```python
from build123d import *

# Parameters (mm, degrees)
SKETCH_1_R          = 80
EXTRUDE_1_DEPTH     = 10
SKETCH_2_R          = 10
CUT_EXTRUDE_1_DEPTH = 10
SKETCH_3_R          = 45
EXTRUDE_2_DEPTH     = 140
SKETCH_6_R          = 10
CUT_EXTRUDE_3_DEPTH = 181
SKETCH_7_R          = 30
SKETCH_7_R_2        = 15
EXTRUDE_3_DEPTH     = 60
SKETCH_8_R          = 15
CUT_EXTRUDE_4_DEPTH = 45
SKETCH_9_R          = 10
CUT_EXTRUDE_5_DEPTH = 200
FILLET_1_R          = 2


with BuildPart() as part:
    # 草图1 → 凸台-拉伸1 (new body)
    with BuildSketch(Plane.XY):
        Circle(SKETCH_1_R)
    extrude(amount=EXTRUDE_1_DEPTH)

    # 草图2 → 切除-拉伸1 (cut)
    with BuildSketch(Plane.XY):
        with Locations((32.5, 56.291651246)):
            Circle(SKETCH_2_R)
        with Locations((-32.5, -56.291651246)):
            Circle(SKETCH_2_R)
        with Locations((-65, 0)):
            Circle(SKETCH_2_R)
        with Locations((-32.5, 56.291651246)):
            Circle(SKETCH_2_R)
        with Locations((65, 0)):
            Circle(SKETCH_2_R)
        with Locations((32.5, -56.291651246)):
            Circle(SKETCH_2_R)
    extrude(amount=CUT_EXTRUDE_1_DEPTH, mode=Mode.SUBTRACT)

    # 草图3 → 凸台-拉伸2 (add)
    with BuildSketch(Plane.XY):
        Circle(SKETCH_3_R)
    extrude(amount=-EXTRUDE_2_DEPTH)

    # 草图6 → 切除-拉伸3 (cut, through all)
    with BuildSketch(Plane.XY):
        Circle(SKETCH_6_R)
    extrude(amount=-CUT_EXTRUDE_3_DEPTH, mode=Mode.SUBTRACT)

    # 草图7 → 凸台-拉伸3 (add)
    with BuildSketch(Plane(origin=(0, 0, 0), x_dir=(0, 0, -1), z_dir=(1, 0, 0))):
        with Locations((110, 0)):
            Circle(SKETCH_7_R)
        with Locations((110, 0)):
            Circle(SKETCH_7_R_2, mode=Mode.SUBTRACT)
    extrude(amount=EXTRUDE_3_DEPTH)

    # 草图8 → 切除-拉伸4 (cut, symmetric)
    with BuildSketch(Plane(origin=(0, 0, 0), x_dir=(0, 0, -1), z_dir=(1, 0, 0))):
        with Locations((110, 0)):
            Circle(SKETCH_8_R)
    extrude(amount=CUT_EXTRUDE_4_DEPTH, both=True, mode=Mode.SUBTRACT)

    # 草图9 → 切除-拉伸5 (cut)
    with BuildSketch(Plane.XY.offset(10)):
        Circle(SKETCH_9_R)
    extrude(amount=-CUT_EXTRUDE_5_DEPTH, mode=Mode.SUBTRACT)

    # 圆角1
    fillet_1_edges = [part.edges().sort_by_distance(p)[0] for p in [
        (-80, 0, 0),
        (-80, 0, 10),
    ]]
    fillet(fillet_1_edges, radius=FILLET_1_R)


solid = part.part
```
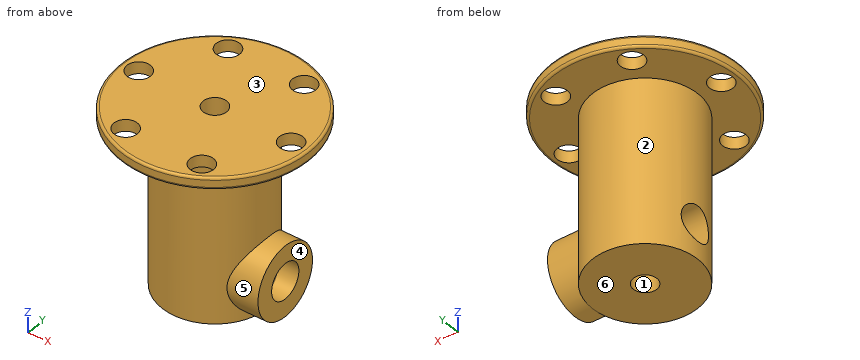
Geometry check sheet. Reference: the model listing, model coordinates, mm. Face numbers are marked on the shaded views. A direction names the side the tool comes from. Give positions to 0.01 mm unless a question says otherwise; leave off trailing zeros. Loops run counter-clockwise (first coordinate to the right, second up) from the corner with the lowest first, then second, coordinate; pieces in that order, holes last. Notation, with made-up numbers: M 45,1 L 56,1 A26 cw 56,31 Z; hole C 22.25,-11.5 d3. An arc over 180 degrees is marked long. Write item = value, one per line.
(1) Tool access check on the marked faces 4, 5 and 6. Record the directions out of +Z, -Z, +X, -X, +Y, -Y that give a thin tool (end or side, any length) a straight path to the whole face; none if there is none.
Answer below:
face_4 = -Z, +X, +Y, -Y
face_5 = +X
face_6 = -Z, +X, -X, +Y, -Y
(2) Release check for a two-part mould opening along Z. For the marked faces 1, 2 and 3 record: released by +Z, released by -Z, zero draft, split by the parting line, or undercut.
Answer below:
face_1 = zero draft
face_2 = undercut
face_3 = released by +Z
(3) Material ranges on line 1 (X direction, y = 0, z = -52); line 2 (Y direction, x = 27.5, z = -120.5); line 3 (Z direction, x = -9, y = 6.5), recorded low to high. Write a range as [from, to].
Answer below:
line_1 = [-45, -10], [10, 45]
line_2 = [-35.62, -10.71], [10.71, 35.62]
line_3 = [-140, -123.52], [-96.48, 10]
(4) Sectioned sample at B-B, the plane z = -90. Record the cut outline in (x, y).
Answer below:
outline = M 39.05,-22.36 L 60,-22.36 L 60,22.36 L 39.05,22.36 A45 ccw long Z; hole C 0,0 d20
(5) Gauge pin test, flat ends, axial feed: pin 1 Ø23 at (x, y) = (32.5, 56.29) entering from -Z; pin 2 Ø4 at (x, z) = (-20, -12) entering from -Y; pin 3 Ø12 at (x, z) = (-44, -76.5) entering from +Y. Record the tip position at first contact, or that the pin passes through.
Answer below:
pin_1 = 0
pin_2 = -41.24
pin_3 = 24.1
(6) Sectioned sample at D-D, the plane y = 51. State how many separate pieces and enclosed holes the cut face has, plus the area to 3 significant figures.
Answer below:
separate_pieces = 3
enclosed_holes = 0
area = 889 mm2
(7) Sectioned sample at C-C, the plane z = -110. Record the cut outline in (x, y).
Answer below:
outline = M -42.43,-15 A45 ccw 33.54,-30 L 60,-30 L 60,-15 Z; M -42.43,15 L 60,15 L 60,30 L 33.54,30 A45 ccw Z
(8) Sectioned sample at A-A, the plane x = 0. Record the cut outline in (y, z), plus the area to 3 significant figures.
Answer below:
outline = M -80,2 A2 ccw -78,0 L -45,0 L -45,-140 L -10,-140 L -10,-121.18 A15 cw -10,-98.82 L -10,10 L -78,10 A2 ccw -80,8 Z; M 10,-140 L 45,-140 L 45,0 L 78,0 A2 ccw 80,2 L 80,8 A2 ccw 78,10 L 10,10 L 10,-98.82 A15 cw 10,-121.18 Z
area = 11,000 mm2
